```python
from build123d import *

# Parameters (mm, degrees)
F0_R     = 4
F0_R_2   = 2
F1_DEPTH = 8.5
F2_R     = 6.5
F3_DEPTH = 2
F4_DEPTH = 3


with BuildPart() as f1:
    # F0 (on Top) → F1 (new body)
    with BuildSketch(Plane.XY):
        Circle(F0_R)
        Circle(F0_R_2, mode=Mode.SUBTRACT)
    extrude(amount=F1_DEPTH)

    # F2 (on Top) → F3 (join)
    with BuildSketch(Plane.XY):
        Circle(F2_R)
    extrude(amount=-F3_DEPTH)

    # F0 (on Top) → F4 (cut)
    with BuildSketch(Plane.XY):
        Circle(F0_R_2)
    extrude(amount=-F4_DEPTH, mode=Mode.SUBTRACT)


solid = f1.part
```
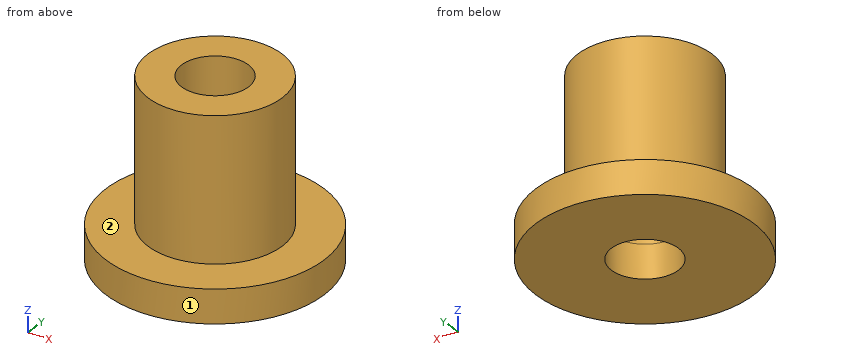
Geometry check sheet. Reference: the model listing, model coordinates, mm. Face numbers are marked on the shaded views. A direction names the side the tool comes from. Coordinates: 2 decimals unless noted, no trailing zeros. Order: outer loops, then holes, each group sorted by start corner. A loop starts at its lowest first (then second) coordinate and runs counter-clockwise, first axis right, second up. Notation, with made-up numbers: (-25, 12.5) - (-14, 12.5) arc R16 cw to (-14, 25.5) - close; hole circle Ø5 at (-28, 13.5). An arc over 180 degrees is marked (long way). Answer in a Markdown table with one row per item. Add a question column.
1. Section check C-C (z = 4.25). Enter the section's corners in (x, y), plus the area to 3 significant figures.
2. Section check D-D (x = 5). Enter the section's corners in (y, z), plus the area to 3 significant figures.
3. Gauge pin test, flat ends, axial feed: pin 1 Ø1.5 at (y, z) = (-3, 1) entering from -X; pin 2 Ø4 at (x, z) = (-4, 4) entering from -Y; pin 3 Ø4 at (y, z) = (0, 4.5) entering from -X. Record the tip position at first contact, or that the pin passes through.
4. Material ranges on L1, parallel to Y at x = 0, z = -0.9; L2, parallel to Y at x = 0, z = 4.75; L3, parallel to Z at x = -4, y = 1.25, recorded low to high. Write a range as [from, to].
5. Access from +Z, -Z, +X, -X, +Y, -Y to the whole of each face (thin tool, end or side, straight path). Record for the marked faces 1 and 2.
6. Section check A-A (x = 0). Enter the section's corners in (y, z).
Data:
| question | item | result |
|---|---|---|
| 1 | outline | circle Ø8 at (0, 0); hole circle Ø4 at (0, 0) |
| 1 | area | 37.7 mm² |
| 2 | outline | (-4.15, -2) - (4.15, -2) - (4.15, 0) - (-4.15, 0) - close |
| 2 | area | 16.6 mm² |
| 3 | pin 1 | stops at x = -3.31 |
| 3 | pin 2 | stops at y = -3.46 |
| 3 | pin 3 | stops at x = -4 |
| 4 | L1 | y = [-6.5, -2], [2, 6.5] |
| 4 | L2 | y = [-4, -2], [2, 4] |
| 4 | L3 | z = [-2, 0] |
| 5 | face 1 | +Z, -Z |
| 5 | face 2 | +Z |
| 6 | outline | (-6.5, -2) - (-2, -2) - (-2, 8.5) - (-4, 8.5) - (-4, 0) - (-6.5, 0) - close; (2, -2) - (6.5, -2) - (6.5, 0) - (4, 0) - (4, 8.5) - (2, 8.5) - close |
